Here's how the part is built. I have some questions about the finished solid (model axes, mm). Face numbers are marked on the shaded views. A direction names the side the tool comes from. Round coordinates to 2 decimals unless told otherwise and drop trailing zeros. Loops run counter-clockwise (first coordinate to the right, second up) from the corner with the lowest first, then second, coordinate; pieces in that order, holes last. Notation, with made-up numbers: (-32, -12) - (22, -12) arc R15 ccw to (22, 15) - close; hole circle Ø2 at (51.25, 5). An arc over 180 degrees is marked (long way). Answer as a JSON object with one key per item and string values. Group by question number.
1) Which directions (+Z, -Z, +X, -X, +Y, -Y) give clear straight access to the entire face, cutting with the end or side of a thin tool? Please do the marked faces 5, 6, 7 and 8.
2) I want a section at A-A, the plane y = 26. Please give me the cut outline in (x, z) (3 decimals).
3) I want a section at B-B, the plane z = 30. Please give me the cut outline in (x, y), then the cut area to 3 significant figures.
4) I want a section at D-D, the plane z = 4. Please give me the cut outline in (x, y), then the cut area to 3 significant figures.
5) If I drill on line 1 along X through (y, z) = (32.5, 14.5); line 2 along X through (y, z) = (19, 21); line 3 along X through (y, z) = (16, 11.5), over which ranges is the centre line in solid material (lowest first)? Write a range as [from, to].
6) If we mould it in two halves opening along Y, with no side actions, what happens to the marked faces 1, 2, 3 and 4? For each: pulls with the +Y half, pulls with the -Y half, needs draft (parallel to the pull), parting line crosses it, or undercut.
7) Will these pins go through, and if not, where does the flat tip stop? P1, Ø10, axis at y = 27.5, z = 7, coming from the +X side; P2, Ø1.4, axis at x = 22.5, y = 20, coming from the -Z side (3 decimals); P3, Ø10, axis at x = 10.5, z = 21.5, coming from the -Y side.
from build123d import *

# Parameters (mm, degrees)
F0_W      = 38.1
F0_H      = 38.1
F1_DEPTH  = 38.1
F6_DEPTH  = 38.1
F8_DEPTH  = 38.1
F9_W      = 7.62
F9_H      = 25.4
F10_DEPTH = 38.1


with BuildPart() as f1:
    # F0 (on Right) → F1 (new body)
    with BuildSketch(Plane.YZ):
        with Locations((19.05, 19.05)):
            Rectangle(F0_W, F0_H)
    extrude(amount=F1_DEPTH)

    # F5 (on offset) → F6 (cut)
    with BuildSketch(Plane.XZ.offset(-38.1)):
        Polygon((38.1, 0), (38.1, 38.1), (31.75, 0), align=None)
        Polygon((31.75, 38.1), (6.35, 38.1), (11.43, 15.875), (16.51, 28.575), (21.59, 28.575), (26.67, 15.875), align=None)
        Polygon((19.05, 15.875), (12.7, 0), (25.4, 0), align=None)
        Polygon((0, 38.1), (0, 0), (6.35, 0), align=None)
    extrude(amount=F6_DEPTH, mode=Mode.SUBTRACT)

    # F7 (on offset) → F8 (cut)
    with BuildSketch(Plane.YZ.offset(38.1)):
        Polygon((0, 38.1), (0, 0), (6.35, 38.1), align=None)
        Polygon((25.4, 38.1), (12.7, 38.1), (19.05, 22.225), align=None)
        Polygon((31.75, 38.1), (38.1, 0), (38.1, 38.1), align=None)
        Polygon((11.43, 22.225), (6.35, 0), (31.75, 0), (26.67, 22.225), (21.59, 9.525), (16.51, 9.525), align=None)
    extrude(amount=-F8_DEPTH, mode=Mode.SUBTRACT)

    # F9 (on offset) → F10 (cut)
    with BuildSketch(Plane.XY.offset(38.1)):
        with Locations((26.67, 12.7)):
            Rectangle(F9_W, F9_H)
        Polygon((15.24, 38.1), (7.62, 38.1), (7.62, 12.7), (15.24, 12.594295), align=None)
    extrude(amount=-F10_DEPTH, mode=Mode.SUBTRACT)


solid = f1.part
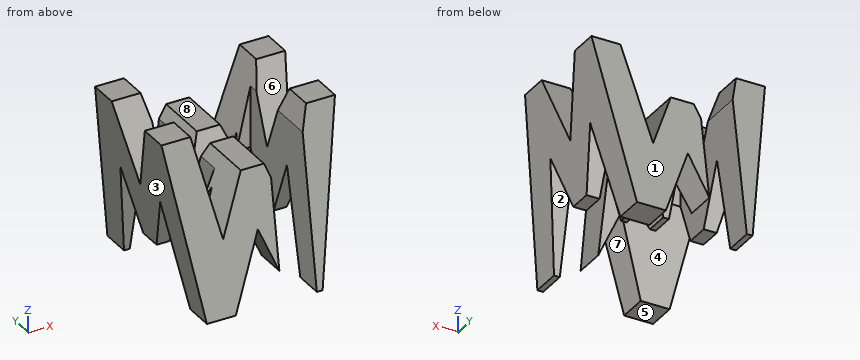
Outcome:
{
 "1": {"face 5": "-Z, +X, -X, +Y, -Y", "face 6": "+Z, +X, -X", "face 7": "-Z, +Y, -Y", "face 8": "+Z, +Y, -Y"},
 "2": {"outline": "(0, 38.1) - (2.925, 20.55) - (7.62, 20.55) - (7.62, 32.544) - (6.35, 38.1) - close; (15.24, 20.55) - (24.8, 20.55) - (21.59, 28.575) - (16.51, 28.575) - (15.24, 25.4) - close; (27.739, 20.55) - (35.175, 20.55) - (38.1, 38.1) - (31.75, 38.1) - close"},
 "3": {"outline": "(1.35, 5) - (8.2, 5) - (8.2, 12.69) - (7.62, 12.7) - (7.62, 15.94) - (1.35, 15.94) - close; (1.35, 22.16) - (7.62, 22.16) - (7.62, 33.1) - (1.35, 33.1) - close; (29.9, 25.4) - (30.48, 25.4) - (30.48, 22.16) - (36.75, 22.16) - (36.75, 33.1) - (29.9, 33.1) - close; (30.48, 5) - (36.75, 5) - (36.75, 15.94) - (30.48, 15.94) - close", "area": "283 mm^2"},
 "4": {"outline": "(5.68, 0.67) - (14.3, 0.67) - (14.3, 7.26) - (5.68, 7.26) - close; (5.68, 30.84) - (7.62, 30.84) - (7.62, 37.43) - (5.68, 37.43) - close; (23.8, 30.84) - (32.42, 30.84) - (32.42, 37.43) - (23.8, 37.43) - close; (30.48, 0.67) - (32.42, 0.67) - (32.42, 7.26) - (30.48, 7.26) - close", "area": "139 mm^2"},
 "5": {"line 1": "[3.93, 7.62], [15.24, 18.5], [19.6, 34.17]", "line 2": "[2.85, 7.62], [15.24, 22.86], [30.48, 35.25]", "line 3": "[4.43, 7.62], [15.24, 17.3], [20.8, 22.86], [30.48, 33.67]"},
 "6": {"face 1": "pulls with the +Y half", "face 2": "undercut", "face 3": "needs draft", "face 4": "undercut"},
 "7": {"P1": "x = 33.71", "P2": "z = 9.525", "P3": "y = 2.75"}
}
